from build123d import *

# Parameters (mm, degrees)
SKETCH1_W                                      = 101.6
SKETCH1_H                                      = 57.15
BOSS_EXTRUDE1_DEPTH                            = 6.35
CBORE_FOR_6_SOCKET_HEAD_CAP_SCREW1_D           = 4.3053
CBORE_FOR_6_SOCKET_HEAD_CAP_SCREW1_CBORE_D     = 7.14502
CBORE_FOR_6_SOCKET_HEAD_CAP_SCREW1_CBORE_DEPTH = 3.5052
F_1_4_CLEARANCE_HOLE1_D                        = 7.14248


with BuildPart() as part:
    # Sketch1 → Boss-Extrude1 (new body)
    with BuildSketch(Plane(origin=(0, 0, 0), x_dir=(1, 0, 0), z_dir=(0, 1, 0))):
        with Locations((50.8, -28.575)):
            Rectangle(SKETCH1_W, SKETCH1_H)
    extrude(amount=BOSS_EXTRUDE1_DEPTH)

    # CBORE for #6 Socket Head Cap Screw1 (through all)
    with Locations(Plane(origin=(0, 6.35, 0), x_dir=(1, 0, 0), z_dir=(0, 1, 0))):
        with Locations((14.2875, -44.45), (87.3125, -44.45)):
            CounterBoreHole(CBORE_FOR_6_SOCKET_HEAD_CAP_SCREW1_D / 2, CBORE_FOR_6_SOCKET_HEAD_CAP_SCREW1_CBORE_D / 2, CBORE_FOR_6_SOCKET_HEAD_CAP_SCREW1_CBORE_DEPTH)

    # 1/4 Clearance Hole1 (through all)
    with Locations(Plane(origin=(0, 6.35, 0), x_dir=(1, 0, 0), z_dir=(0, 1, 0))):
        with Locations((19.05, -12.7), (82.55, -12.7)):
            Hole(F_1_4_CLEARANCE_HOLE1_D / 2)


solid = part.part
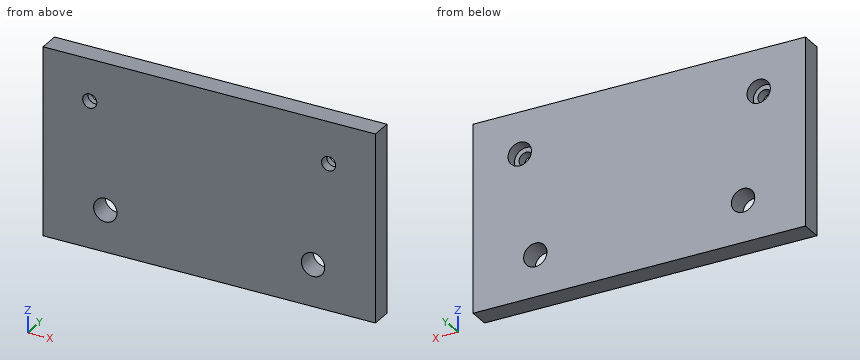
Design review of the part built by this model. Coordinates are the model's own, in mm. Give positions to 0.01 mm unless a question says otherwise; leave off trailing zeros. Order: outer loops, then holes, each group sorted by start corner. A loop starts at its lowest first (then second) coordinate and runs counter-clockwise, first axis right, second up.
1. Add section A-A, the plane x = 19.05. State the section outline as (y, z) points.
Solution:
outline: (0, 0) - (6.35, 0) - (6.35, 9.13) - (0, 9.13) - close; (0, 16.27) - (6.35, 16.27) - (6.35, 57.15) - (0, 57.15) - close
2. Add section B-B, the plane y = 4.75. State the section outline as (x, z) points, then the cut area to 3 significant figures.
Solution:
outline: (0, 0) - (101.6, 0) - (101.6, 57.15) - (0, 57.15) - close; hole circle Ø7.15 at (14.29, 44.45); hole circle Ø7.14 at (19.05, 12.7); hole circle Ø7.14 at (82.55, 12.7); hole circle Ø7.15 at (87.31, 44.45)
area: 5,650 mm2
3. Add section C-C, the plane z = 12.7. State the section outline as (x, y) points.
Solution:
outline: (0, 0) - (15.48, 0) - (15.48, 6.35) - (0, 6.35) - close; (22.62, 0) - (78.98, 0) - (78.98, 6.35) - (22.62, 6.35) - close; (86.12, 0) - (101.6, 0) - (101.6, 6.35) - (86.12, 6.35) - close
4. To check wall thickness, follow L1, parallel to X at y = 3.85, z = 44.45 (3 decimals); L2, parallel to X at y = 5.25, z = 12.7; L3, parallel to Z at x = 19.05, y = 3.75. State the ranges of each line that lie inside material, in increasing order.
Solution:
L1: x = 0 to 10.715, 17.86 to 83.74, 90.885 to 101.6
L2: x = 0 to 15.48, 22.62 to 78.98, 86.12 to 101.6
L3: z = 0 to 9.13, 16.27 to 57.15
5. Add section D-D, the plane z = 43.5. State the section outline as (x, y) points.
Solution:
outline: (0, 0) - (12.36, 0) - (12.36, 2.84) - (10.84, 2.84) - (10.84, 6.35) - (0, 6.35) - close; (16.22, 0) - (85.38, 0) - (85.38, 2.84) - (83.87, 2.84) - (83.87, 6.35) - (17.73, 6.35) - (17.73, 2.84) - (16.22, 2.84) - close; (89.24, 0) - (101.6, 0) - (101.6, 6.35) - (90.76, 6.35) - (90.76, 2.84) - (89.24, 2.84) - close
6. For pin 1 Ø4.5 at (x, z) = (87.31, 44.45) entering from +Y, flat-tipped, find the tip position at first contact; note if it passes through.
Solution:
pin 1: stops at y = 2.84
